```python
from build123d import *

# Parameters (mm, degrees)
F1_DEPTH = 25.4
F2_W     = 10.16
F2_H     = 7.62
F3_DEPTH = 12.7
F4_R     = 5.08


with BuildPart() as f1:
    # F0 (on Top) → F1 (new body)
    with BuildSketch(Plane.XY):
        with BuildLine():
            ThreePointArc((0, 19.05), (19.05, 0), (0, -19.05))
            Line((0, -19.05), (88.9, -19.05))
            Line((88.9, -19.05), (88.9, 19.05))
            Line((88.9, 19.05), (0, 19.05))
        make_face()
    extrude(amount=F1_DEPTH)

    # F2 (on face) → F3 (cut)
    with BuildSketch(Plane.XY.offset(25.4)):
        with Locations((31.75, 0)):
            Rectangle(F2_W, F2_H)
    extrude(amount=-F3_DEPTH, mode=Mode.SUBTRACT)

    # F4
    f4_edges = [f1.edges().sort_by_distance(p)[0] for p in [
        (44.45, -19.05, 25.4),
        (44.45, 19.05, 25.4),
        (44.45, 19.05, 0),
        (44.45, -19.05, 0),
        (88.9, -19.05, 12.7),
        (88.9, 19.05, 12.7),
        (88.9, 0, 0),
        (88.9, 0, 25.4),
    ]]
    fillet(f4_edges, radius=F4_R)


solid = f1.part
```
Check sheet for the modelled part. Datum: model origin and axes. Units: mm. A direction names the side the tool comes from. Round coordinates to 2 decimals unless told otherwise and drop trailing zeros. Loops run counter-clockwise (first coordinate to the right, second up) from the corner with the lowest first, then second, coordinate; pieces in that order, holes last. Notation, with made-up numbers: (6, 69.5) -> (46, 69.5) arc R16 ccw to (46, 89.5) -> close; hole circle Ø6 at (55, -28.75). An arc over 180 degrees is marked (long way). Answer in a Markdown table with one row per item.
Q1. Sectioned sample at C-C on y = 0. Enter the section's corners in (x, z).
Data:
| item | result |
|---|---|
| outline | (19.05, 0) -> (83.82, 0) arc R5.08 ccw to (88.9, 5.08) -> (88.9, 20.32) arc R5.08 ccw to (83.82, 25.4) -> (36.83, 25.4) -> (36.83, 12.7) -> (26.67, 12.7) -> (26.67, 25.4) -> (19.05, 25.4) -> close |
Q2. Set-up check for faces 1 (the face through (26.67, 0, 19)), 2 (the face through (19.045, 0.419, 12.522)): record each of +Z, -Z, +X, -X, +Y, -Y from which the full face is reachable in a straight line by a thin tool's end or side.
Data:
| item | result |
|---|---|
| face 1 | +Z |
| face 2 | +Z, -Z, -X |
Q3. Sectioned sample at D-D on x = 67.5. Enter the section's corners in (y, z), then the cut area to 3 significant figures.
Data:
| item | result |
|---|---|
| outline | (-19.05, 5.08) arc R5.08 ccw to (-13.97, 0) -> (13.97, 0) arc R5.08 ccw to (19.05, 5.08) -> (19.05, 20.32) arc R5.08 ccw to (13.97, 25.4) -> (-13.97, 25.4) arc R5.08 ccw to (-19.05, 20.32) -> close |
| area | 946 mm^2 |
Q4. Sectioned sample at A-A on x = 15. Enter the section's corners in (y, z), then the cut area to 3 significant figures.
Data:
| item | result |
|---|---|
| outline | (-19.05, 5.08) arc R5.08 ccw to (-13.97, 0) -> (-11.74, 0) -> (-11.74, 25.4) -> (-13.97, 25.4) arc R5.08 ccw to (-19.05, 20.32) -> close; (11.74, 0) -> (13.97, 0) arc R5.08 ccw to (19.05, 5.08) -> (19.05, 20.32) arc R5.08 ccw to (13.97, 25.4) -> (11.74, 25.4) -> close |
| area | 349 mm^2 |
Q5. Release check for a two-part mould opening along X. For faces 3 (the face through (41, -19.05, 13)), 4 (the face through (87.372, 0.196, 1.449)), 5 (the face through (32, 3.81, 19)) record: released by +X, released by -X, zero draft, split by the parting line, or undercut.
Data:
| item | result |
|---|---|
| face 3 | zero draft |
| face 4 | released by +X |
| face 5 | undercut |
Q6. Thickness scan on L1, parallel to Y at x = 63, z = 5; L2, parallel to Y at x = 12, z = 10; L3, parallel to X at y = 0.5, z = 21.25. Record the ranges inside material, lowest first.
Data:
| item | result |
|---|---|
| L1 | y = -19.05 to 19.05 |
| L2 | y = -19.05 to -14.8, 14.8 to 19.05 |
| L3 | x = 19.04 to 26.67, 36.83 to 88.81 |
Q7. Go/stop test with flat-tipped pins: P1, Ø2.5, axis at x = 29.5, y = 0, coming from the +Z side; P2, Ø4, axis at y = 1.5, z = 20, coming from the -X side; P3, Ø3, axis at y = -3, z = 3.5, coming from the -X side; P4, Ø3, axis at y = 1.5, z = 21.5, coming from the +X side. Record where each tip stops, or that it passes through.
Data:
| item | result |
|---|---|
| P1 | stops at z = 12.7 |
| P2 | stops at x = 18.73 |
| P3 | stops at x = 18.51 |
| P4 | stops at x = 88.9 |
Q8. Sectioned sample at B-B on z = 19. Enter the section's corners in (x, y).
Data:
| item | result |
|---|---|
| outline | (0, -19.05) -> (83.82, -19.05) arc R5.08 ccw to (88.9, -13.97) -> (88.9, 13.97) arc R5.08 ccw to (83.82, 19.05) -> (0, 19.05) arc R19.05 cw to start; hole (26.67, -3.81) -> (36.83, -3.81) -> (36.83, 3.81) -> (26.67, 3.81) -> close |
